Can you work these out from the model? Positions are in its coordinate system, mm. A direction names the side the tool comes from. Give positions to 0.01 mm unless a question says otherwise; leave off trailing zeros. Loops run counter-clockwise (first coordinate to the right, second up) from the corner with the lowest first, then second, coordinate; pieces in that order, holes last. Notation, with made-up numbers: M 77,54 L 120,54 A12 cw 120,58 Z; hole C -22.5,0 d2. An arc over 180 degrees is marked long. Answer as a JSON object with one key per item and string values.
```python
from build123d import *

# Parameters (mm, degrees)
SKETCH_W                        = 30
SKETCH_H                        = 72
SKETCH_R                        = 1.75
PAD_DEPTH                       = 24
SKETCH001_W                     = 26
SKETCH001_H                     = 42
POCKET_DEPTH                    = 21
POCKET001_DEPTH                 = 21
POCKET001_LINEARPATTERN_2_DEPTH = 21
POCKET001_LINEARPATTERN_3_DEPTH = 21
POCKET001_LINEARPATTERN_4_DEPTH = 21
POCKET001_LINEARPATTERN_5_DEPTH = 21
POCKET001_LINEARPATTERN_6_DEPTH = 21
SKETCH005_R                     = 2
POCKET002_DEPTH                 = 7.5
PAD003_DEPTH                    = 17
PAD003_DEPTH_BACK               = 17
POCKET004_DEPTH                 = 29.001


with BuildPart() as part:
    # Sketch → Pad (new body)
    with BuildSketch(Plane.XY):
        Rectangle(SKETCH_W, SKETCH_H)
        with Locations((0, 18)):
            Circle(SKETCH_R, mode=Mode.SUBTRACT)
        with Locations((0, -8)):
            Circle(SKETCH_R, mode=Mode.SUBTRACT)
    extrude(amount=PAD_DEPTH)

    # Sketch001 → Pocket (cut)
    with BuildSketch(Plane.XY.offset(24)):
        with Locations((0, 5)):
            Rectangle(SKETCH001_W, SKETCH001_H)
    extrude(amount=-POCKET_DEPTH, mode=Mode.SUBTRACT)

    # Sketch002 → Pocket001 (cut)
    with BuildSketch(Plane.XY.offset(24)):
        Polygon((-18.773503, 16), (-13, 26), (-11.5, 26), (-17.273503, 16), align=None)
    pocket001 = extrude(amount=-POCKET001_DEPTH, mode=Mode.SUBTRACT)

    # Sketch002 LinearPattern 2 → Pocket001 LinearPattern 2 (cut)
    with BuildSketch(Plane(origin=(0, -8.4, 24), x_dir=(1, 0, 0), z_dir=(0, 0, 1))):
        Polygon((-18.773503, 16), (-13, 26), (-11.5, 26), (-17.273503, 16), align=None)
    pocket001_linearpattern_2 = extrude(amount=-POCKET001_LINEARPATTERN_2_DEPTH, mode=Mode.SUBTRACT)

    # Sketch002 LinearPattern 3 → Pocket001 LinearPattern 3 (cut)
    with BuildSketch(Plane(origin=(0, -16.8, 24), x_dir=(1, 0, 0), z_dir=(0, 0, 1))):
        Polygon((-18.773503, 16), (-13, 26), (-11.5, 26), (-17.273503, 16), align=None)
    pocket001_linearpattern_3 = extrude(amount=-POCKET001_LINEARPATTERN_3_DEPTH, mode=Mode.SUBTRACT)

    # Sketch002 LinearPattern 4 → Pocket001 LinearPattern 4 (cut)
    with BuildSketch(Plane(origin=(0, -25.2, 24), x_dir=(1, 0, 0), z_dir=(0, 0, 1))):
        Polygon((-18.773503, 16), (-13, 26), (-11.5, 26), (-17.273503, 16), align=None)
    pocket001_linearpattern_4 = extrude(amount=-POCKET001_LINEARPATTERN_4_DEPTH, mode=Mode.SUBTRACT)

    # Sketch002 LinearPattern 5 → Pocket001 LinearPattern 5 (cut)
    with BuildSketch(Plane(origin=(0, -33.6, 24), x_dir=(1, 0, 0), z_dir=(0, 0, 1))):
        Polygon((-18.773503, 16), (-13, 26), (-11.5, 26), (-17.273503, 16), align=None)
    pocket001_linearpattern_5 = extrude(amount=-POCKET001_LINEARPATTERN_5_DEPTH, mode=Mode.SUBTRACT)

    # Sketch002 LinearPattern 6 → Pocket001 LinearPattern 6 (cut)
    with BuildSketch(Plane(origin=(0, -42, 24), x_dir=(1, 0, 0), z_dir=(0, 0, 1))):
        Polygon((-18.773503, 16), (-13, 26), (-11.5, 26), (-17.273503, 16), align=None)
    pocket001_linearpattern_6 = extrude(amount=-POCKET001_LINEARPATTERN_6_DEPTH, mode=Mode.SUBTRACT)

    # Mirrored: Pocket001, Pocket001 LinearPattern 2, Pocket001 LinearPattern 3, Pocket001 LinearPattern 4, Pocket001 LinearPattern 5, Pocket001 LinearPattern 6 across Sketch002 V_Axis
    add(pocket001.mirror(Plane(origin=(0, 0, 24), x_dir=(0, 0, 1), z_dir=(1, 0, 0))), mode=Mode.SUBTRACT)
    add(pocket001_linearpattern_2.mirror(Plane(origin=(0, 0, 24), x_dir=(0, 0, 1), z_dir=(1, 0, 0))), mode=Mode.SUBTRACT)
    add(pocket001_linearpattern_3.mirror(Plane(origin=(0, 0, 24), x_dir=(0, 0, 1), z_dir=(1, 0, 0))), mode=Mode.SUBTRACT)
    add(pocket001_linearpattern_4.mirror(Plane(origin=(0, 0, 24), x_dir=(0, 0, 1), z_dir=(1, 0, 0))), mode=Mode.SUBTRACT)
    add(pocket001_linearpattern_5.mirror(Plane(origin=(0, 0, 24), x_dir=(0, 0, 1), z_dir=(1, 0, 0))), mode=Mode.SUBTRACT)
    add(pocket001_linearpattern_6.mirror(Plane(origin=(0, 0, 24), x_dir=(0, 0, 1), z_dir=(1, 0, 0))), mode=Mode.SUBTRACT)

    # SubtractivePipe: sweep along a path in Sketch003
    with BuildLine(Plane.XY.offset(24)) as subtractivepipe_path:
        Line((-9, -16), (-9, -22))
        ThreePointArc((-9, -22), (-5.799746, -26.924429), (0, -26))
        ThreePointArc((0, -26), (5.799746, -25.075571), (9, -30))
        Line((9, -30), (9, -36))
    # Sketch004 → SubtractivePipe (sweep, cut)
    with BuildSketch(Plane.XZ.offset(36)):
        with BuildLine():
            Line((6.5, 24), (6.5, 12))
            ThreePointArc((6.5, 12), (9, 9.5), (11.5, 12))
            Line((11.5, 12), (11.5, 24))
            Line((11.5, 24), (6.5, 24))
        make_face()
    sweep(path=subtractivepipe_path.line, mode=Mode.SUBTRACT)

    # Sketch005 → Pocket002 (cut)
    with BuildSketch(Plane.XY.offset(24)):
        with Locations((-10, -31)):
            Circle(SKETCH005_R)
        with Locations((8, 31)):
            Circle(SKETCH005_R)
    extrude(amount=-POCKET002_DEPTH, mode=Mode.SUBTRACT)

    # Sketch010 → Pad003 (join, two sides)
    with BuildSketch(Plane(origin=(0, 36, 0), x_dir=(0, 1, 0), z_dir=(1, 0, 0))) as pad003_sk:
        Polygon((0, 0), (0, 29), (12, 0), align=None)
    extrude(amount=PAD003_DEPTH)
    extrude(pad003_sk.sketch, amount=-PAD003_DEPTH_BACK)

    # Sketch011 → Pocket004 (cut, through all)
    with BuildSketch(Plane.XY):
        Polygon((-17, 36), (-6, 54), (6, 54), (17, 36), (17, 56), (-17, 56), align=None)
    extrude(amount=POCKET004_DEPTH, mode=Mode.SUBTRACT)


solid = part.part
```
1) Suppose I cut it at D-D, the plane y = -17. Write out the boundary of the cut face in (x, z), and give its area (3 significant figures).
Answer list:
{"outline": "M -15,0 L 15,0 L 15,24 L 13.58,24 L 13.58,3 L 12.08,3 L 12.08,24 L -6.5,24 L -6.5,12 A2.5 cw -11.5,12 L -11.5,24 L -12.08,24 L -12.08,3 L -13.58,3 L -13.58,24 L -15,24 Z", "area": "587 mm^2"}
2) Suppose I cut it at C-C, the plane y = 4.5. Write out the boundary of the cut face in (x, z), and give its area (3 significant figures).
Answer list:
{"outline": "M -15,0 L 15,0 L 15,3 L 14.21,3 L 14.21,24 L 13,24 L 13,3 L -13,3 L -13,24 L -14.21,24 L -14.21,3 L -15,3 Z", "area": "141 mm^2"}
3) Please list where these lines run through material, in increasing order: line 1 along Y through (x, z) = (-10, 19.5); line 2 along Y through (x, z) = (2.5, 17); line 3 along X through (y, z) = (-10.5, 16.75). Write a range as from..to.
Answer list:
{"line 1": "-36..-33, -29..-26.63, 26..39.93", "line 2": "-36..-27.33, -22.19..-16, 26..40.97", "line 3": "-15..-14.67, -13.17..-13, 13..13.17, 14.67..15"}
4) If we mould it in two halves opening along Y, with no side actions, what happens to faces 1 (the flat face through (11.5, -33, 18)), 2 (the flat face through (-1, 36, 25)), 3 (the flat face through (14.014, 24.244, 13.647))? For each: +Y half, -Y half, draft (parallel to the pull), parting line (faces both ways), or undercut.
Answer list:
{"face 1": "draft", "face 2": "-Y half", "face 3": "undercut"}
5) Will these pins go through, and if not, where does the flat tip stop? pin 1 Ø12 at (x, y) = (9.5, -9.5) entering from +Z; pin 2 Ø6.5 at (y, z) = (-4, 15.5) entering from +X; pin 3 Ø4 at (x, y) = (7.5, -1) entering from +Z.
Answer list:
{"pin 1": "z = 24", "pin 2": "x = 15", "pin 3": "z = 3"}
6) For faces 4 (the flat face through (6.5, -33, 18)), 5 (the flat face through (13, 20, 14)), 6 (the flat face through (-7, -30, 24)), 7 (the flat face through (-15, -1, 12)), which set-ups out of +Z, -Z, +X, -X, +Y, -Y let a thin tool reach every point of the face, with its end or its side?
Answer list:
{"face 4": "+Z, -Y", "face 5": "+Z", "face 6": "+Z, +X, -X, -Y", "face 7": "+Z, -Z, -X, -Y"}
7) Suppose I cut it at A-A, the plane y = 31. Write out the boundary of the cut face in (x, z).
Answer list:
{"outline": "M -15,0 L 15,0 L 15,24 L 10,24 L 10,16.5 L 6,16.5 L 6,24 L -15,24 Z"}
8) Suppose I cut it at B-B, the plane y = -31. Write out the boundary of the cut face in (x, z), and give its area (3 significant figures).
Answer list:
{"outline": "M -15,0 L 15,0 L 15,24 L 11.5,24 L 11.5,12 A2.5 cw 6.5,12 L 6.5,24 L -8,24 L -8,16.5 L -12,16.5 L -12,24 L -15,24 Z", "area": "620 mm^2"}
